```python
from build123d import *

# Parameters (mm, degrees)
SKETCH1_R           = 20
SKETCH1_R_2         = 14
BOSS_EXTRUDE1_DEPTH = 1.5
SKETCH2_W           = 3
SKETCH2_H           = 2
BOSS_EXTRUDE2_DEPTH = 1
CIRPATTERN1_COUNT   = 12


with BuildPart() as part:
    # Sketch1 → Boss-Extrude1 (new body)
    with BuildSketch(Plane(origin=(0, 0, 0), x_dir=(1, 0, 0), z_dir=(0, 1, 0))):
        Circle(SKETCH1_R)
        Circle(SKETCH1_R_2, mode=Mode.SUBTRACT)
    extrude(amount=BOSS_EXTRUDE1_DEPTH)

    # Sketch2 → Boss-Extrude2 (add)
    with BuildSketch(Plane(origin=(0, 1.5, 0), x_dir=(1, 0, 0), z_dir=(0, 1, 0))):
        with Locations((0, 17)):
            Rectangle(SKETCH2_W, SKETCH2_H)
    boss_extrude2 = extrude(amount=BOSS_EXTRUDE2_DEPTH)

    # CirPattern1: Boss-Extrude2 ×12 about axis
    cirpattern1_axis = Axis((0, 0, 0), (0, 1, 0))
    for i in range(1, CIRPATTERN1_COUNT):
        add(boss_extrude2.rotate(cirpattern1_axis, i * 360 / CIRPATTERN1_COUNT))


solid = part.part
```
The model under review builds one solid part; all positions refer to its coordinate system, in mm. A direction names the side the tool comes from. Give positions to 0.01 mm unless a question says otherwise; leave off trailing zeros. Write each loop counter-clockwise with the first axis right and the second up, starting at its lowest first coordinate (ties: lowest second). Pieces come first, ordered by that corner, then holes. Notation, with made-up numbers: (-19, -5.5) -> (2, -5.5) arc R24 ccw to (2, 9.5) -> close; hole circle Ø2 at (75, -37.75). An arc over 180 degrees is marked (long way). Answer in a Markdown table with one row per item.
1) For L1, parallel to Z at x = 0, y = 0.7; L2, parallel to Y at x = 3.5, z = 16.5, list the stretches that pass through material, from the lowest coordinate up. Write a range as [from, to].
Worked answers:
| item | result |
|---|---|
| L1 | [-20, -14], [14, 20] |
| L2 | [0, 1.5] |
2) Add section C-C on y = 0.85. State the section outline as (x, z) points, plus the area to 3 significant figures.
Worked answers:
| item | result |
|---|---|
| outline | circle Ø40 at (0, 0); hole circle Ø28 at (0, 0) |
| area | 641 mm² |
3) Mouldability with a two-part tool opening along Z and no side actions: class faces 5 (the flat face through (0, 2, -18)), 6 (the flat face through (16, 2, 0)), 7 (the flat face through (-13.96, 1.99, 9.79)) as +Z half, -Z half, draft (parallel to the pull), parting line (faces both ways), or undercut.
Worked answers:
| item | result |
|---|---|
| face 5 | -Z half |
| face 6 | undercut |
| face 7 | +Z half |
4) Add section D-D on x = -4.5. State the section outline as (y, z) points.
Worked answers:
| item | result |
|---|---|
| outline | (0, -19.49) -> (1.5, -19.49) -> (1.5, -13.26) -> (0, -13.26) -> close; (0, 13.26) -> (1.5, 13.26) -> (1.5, 19.49) -> (0, 19.49) -> close |
5) Tool access review of faces 1 (the flat face through (1.5, 2, 17)), 2 (the flat face through (7.98, 1.99, -13.87)), 3 (the flat face through (17, 2, 1.5)), 4 (the flat face through (-9.79, 1.99, 13.96)): name each direction out of +Z, -Z, +X, -X, +Y, -Y from which nothing blocks a thin tool from reaching the whole face with its end or side.
Worked answers:
| item | result |
|---|---|
| face 1 | +Z, -Z, +Y |
| face 2 | +Y |
| face 3 | +X, -X, +Y |
| face 4 | -X, +Y |
6) Add section B-B on z = 0. State the section outline as (x, y) points, plus the area to 3 significant figures.
Worked answers:
| item | result |
|---|---|
| outline | (-20, 0) -> (-14, 0) -> (-14, 1.5) -> (-16, 1.5) -> (-16, 2.5) -> (-18, 2.5) -> (-18, 1.5) -> (-20, 1.5) -> close; (14, 0) -> (20, 0) -> (20, 1.5) -> (18, 1.5) -> (18, 2.5) -> (16, 2.5) -> (16, 1.5) -> (14, 1.5) -> close |
| area | 22.0 mm² |
7) Add section A-A on x = 0. State the section outline as (y, z) points, plus the area to 3 significant figures.
Worked answers:
| item | result |
|---|---|
| outline | (0, -20) -> (1.5, -20) -> (1.5, -18) -> (2.5, -18) -> (2.5, -16) -> (1.5, -16) -> (1.5, -14) -> (0, -14) -> close; (0, 14) -> (1.5, 14) -> (1.5, 16) -> (2.5, 16) -> (2.5, 18) -> (1.5, 18) -> (1.5, 20) -> (0, 20) -> close |
| area | 22.0 mm² |
8) Clearance check with flat-ended pins moving along their axes: P1, Ø1, axis at y = 1.5, z = -13, coming from the +X side; P2, Ø0.8, axis at y = 2, z = 0, coming from the -X side; P3, Ø0.8, axis at y = 2, z = -17.5, coming from the -X side; P4, Ø3, axis at x = -12, z = -3, coming from the +Y side. State where each tip first meets the part, or that it passes through.
Worked answers:
| item | result |
|---|---|
| P1 | x = 15.61 |
| P2 | x = -18 |
| P3 | x = -1.5 |
| P4 | through |
